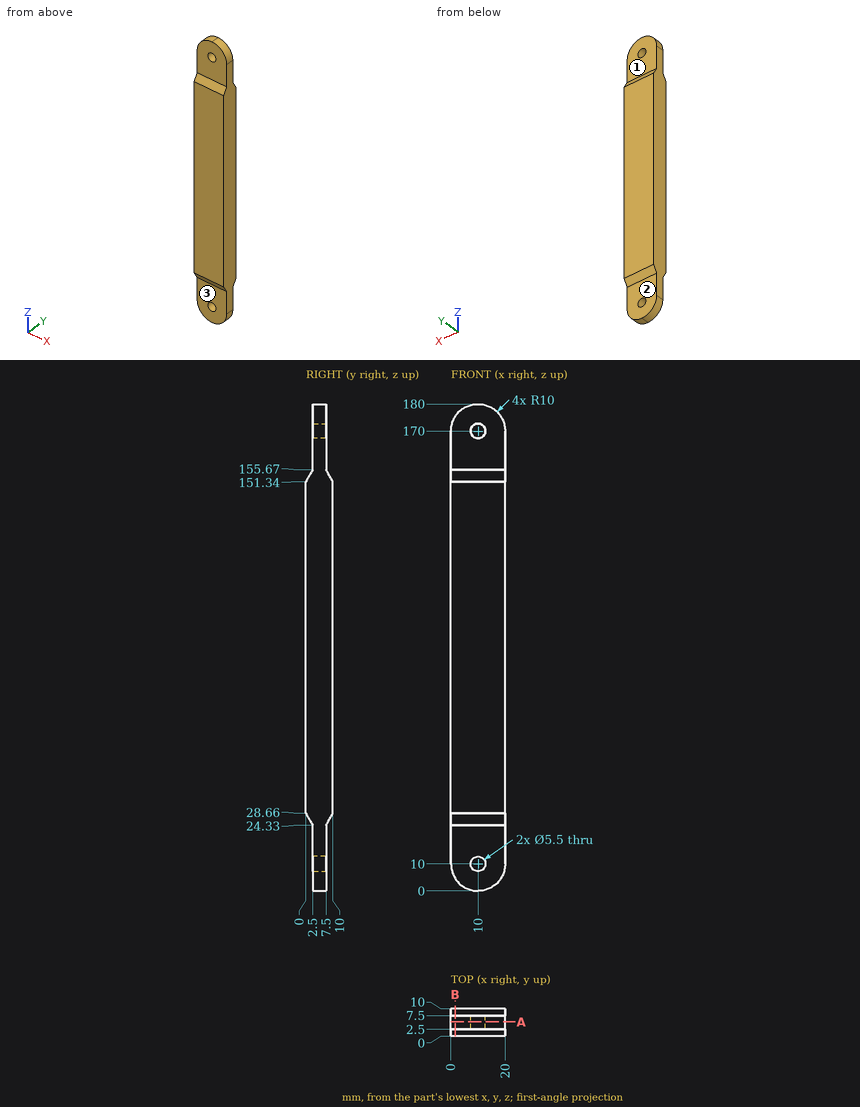
Answer from the drawing. Dimensions are ordinates in mm from the lowest x, y and z of the part. A direction names the side the tool comes from. Coordinates: 2 decimals unless noted, no trailing zeros. Loops run counter-clockwise (first coordinate to the right, second up) from the corner with the lowest first, then second, coordinate; pieces in that order, holes last.
1) For the marked faces 1, 2 and 3, determine the directions among +Z, -Z, +X, -X, +Y, -Y from which every point of the face is accessible in a straight line to the end or side of a thin tool.
Results:
face 1: +Z, +X, -X, +Y
face 2: -Z, +X, -X, +Y
face 3: -Z, +X, -X, -Y
2) Section A-A (y = 5.25) is taken. Give the number of separate pieces and of enclosed holes in the cut face, plus the area to 3 significant figures.
Results:
separate pieces: 1
enclosed holes: 2
area: 3,470 mm2
3) Consider probe 1 along X at (y, z) = (4.55, 10); probe 2 along Y at (x, z) = (7.75, 13.5); probe 3 along X at (y, z) = (5.5, 9). Determine where each line is inside the solid, lowest interval first.
Results:
probe 1: x = 0 to 7.25, 12.75 to 20
probe 2: y = 2.5 to 7.5
probe 3: x = 0.05 to 7.44, 12.56 to 19.95
4) Flat-ended cylindrical pins translate along their axes: pin 1 (6 mm diameter, centred on x = 9, y = 3, fed in from -Z); pin 2 (2 mm diameter, centred on x = 12.5, y = 7, fed in from +Z). Find the tip coordinate at first contact, or state that the pin passes through.
Results:
pin 1: stops at z = 0
pin 2: stops at z = 179.89
5) Section B-B (x = 1.5) is taken. Give the vertices of the cut face in (y, z).
Results:
outline: (0, 28.66) - (2.5, 24.33) - (2.5, 4.73) - (7.5, 4.73) - (7.5, 24.33) - (10, 28.66) - (10, 151.34) - (7.5, 155.67) - (7.5, 175.27) - (2.5, 175.27) - (2.5, 155.67) - (0, 151.34) - close
